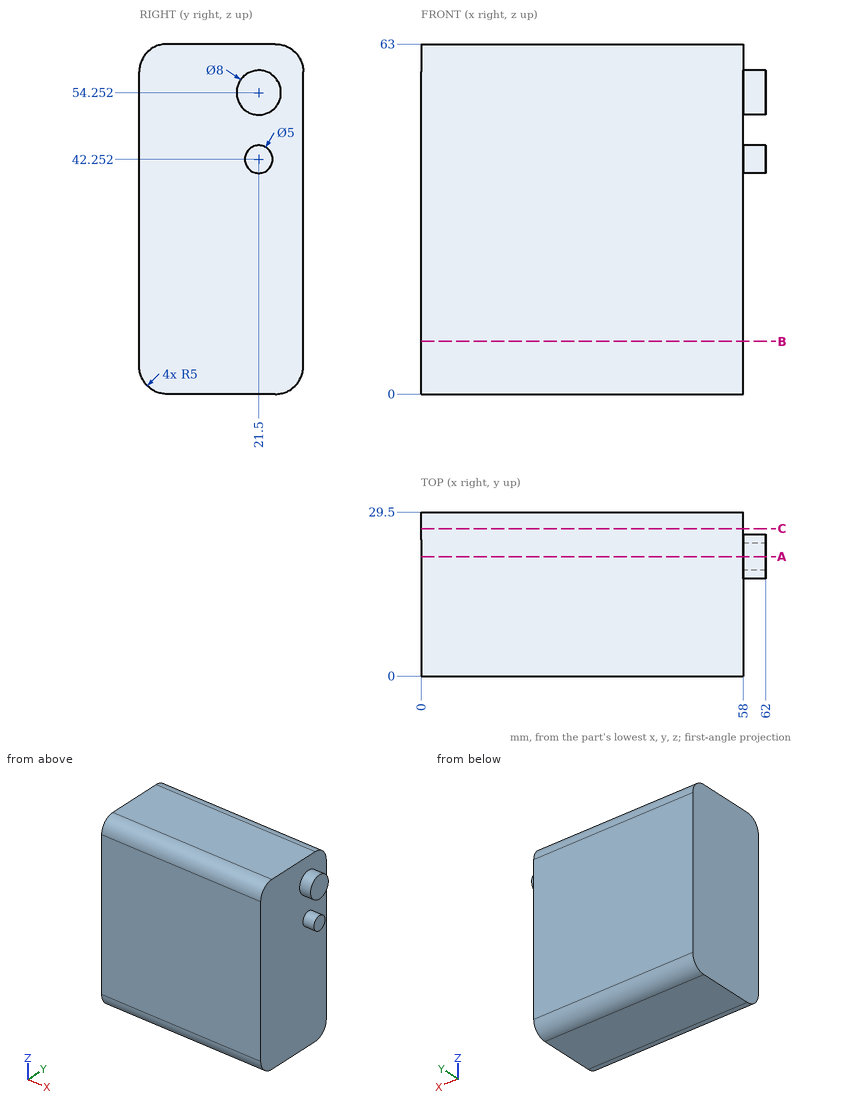
Design review of the part shown in the three views and the two pictorial views. Dimensions are in mm from the part's minimum x, y and z. Give positions to 0.01 mm unless a question says otherwise; leave off trailing zeros. Loops run counter-clockwise (first coordinate to the right, second up) from the corner with the lowest first, then second, coordinate; pieces in that order, holes last. Notation, with made-up numbers: (-3, 76) -> (4, 76) arc R21 ccw to (4, 87) -> close; hole circle Ø10 at (27, -3.75). An arc over 180 degrees is marked (long way). One line per item, written item: value.
Q1. For L1, parallel to X at y = 22.75, z = 45; L2, parallel to Z at x = 51, y = 4.25, list the stretches that pass through material, from the lowest coordinate up.
Numbers:
L1: x = 0 to 58
L2: z = 0.06 to 62.94
Q2. We need section B-B on z = 9.5. Give the boundary of the cut face in (x, y), and give its area (3 significant figures).
Numbers:
outline: (0, 0) -> (58, 0) -> (58, 29.5) -> (0, 29.5) -> close
area: 1,710 mm^2
Q3. We need section C-C on y = 26.5. Give the boundary of the cut face in (x, z), and give its area (3 significant figures).
Numbers:
outline: (0, 0.42) -> (58, 0.42) -> (58, 62.58) -> (0, 62.58) -> close
area: 3,610 mm^2
Q4. For pin 1 Ø8 at (y, z) = (4, 20.5) entering from +X; pin 2 Ø12 at (y, z) = (5, 17) entering from -X, all flat-tipped, find the tip position at first contact; note any pin that passes through.
Numbers:
pin 1: stops at x = 58
pin 2: stops at x = 0
Q5. We need section A-A on y = 21.5. Give the boundary of the cut face in (x, z).
Numbers:
outline: (0, 0) -> (58, 0) -> (58, 39.75) -> (62, 39.75) -> (62, 44.75) -> (58, 44.75) -> (58, 50.25) -> (62, 50.25) -> (62, 58.25) -> (58, 58.25) -> (58, 63) -> (0, 63) -> close
